Study the drawing (mm; zero at the part's minimum x, y, z) and answer. Coordinates: 2 decimals unless noted, no trailing zeros. Write each loop counter-clockwise with the first axis right and the second up, starting at its lowest first coordinate (ties: lowest second). Pieces come first, ordered by that corner, then holes. Notation, with made-up numbers: (74, 42.25) - (125, 42.25) arc R10 cw to (125, 58.25) - close; hole circle Ø1 at (57, -10.5). An arc over 180 degrees is marked (long way). One line per item, written item: value.
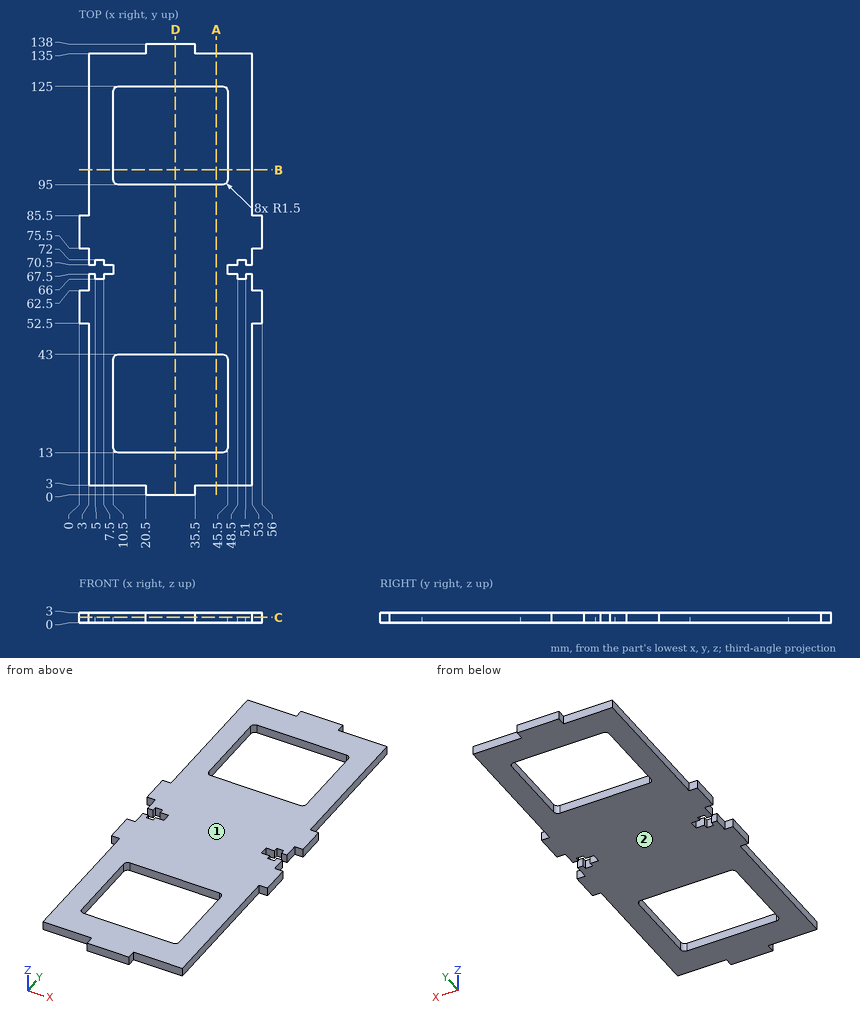
Item 1: Given pin 1 (1.5 mm diameter, centred on x = 55, z = 2, fed in from -Y); pin 2 (1.2 mm diameter, centred on x = 50.5, z = 2, fed in from -Y); pin 3 (1.5 mm diameter, centred on y = 1.5, z = 1, fed in from -X), each flat-ended and moving along its own axis, determine where each tip first touches the part or whether it passes through.
Evaluation:
pin 1: stops at y = 52.5
pin 2: stops at y = 3
pin 3: stops at x = 20.5
Item 2: Section C-C, the plane z = 1.65 is taken. Give the number of separate pieces and of enclosed holes in the cut face, then the cut area to 3 significant figures.
Evaluation:
separate pieces: 1
enclosed holes: 2
area: 4,650 mm2
Item 3: Determine the mould class of the marked faces 1 and 2 for opening direction Z: +Z half, -Z half, draft (parallel to the pull), parting line (faces both ways), or undercut.
Evaluation:
face 1: +Z half
face 2: -Z half
Item 4: Section A-A, the plane x = 42 is taken. Determine the outline of the cut face in (y, z).
Evaluation:
outline: (3, 0) - (13, 0) - (13, 3) - (3, 3) - close; (43, 0) - (95, 0) - (95, 3) - (43, 3) - close; (125, 0) - (135, 0) - (135, 3) - (125, 3) - close
Item 5: Section B-B, the plane y = 99.5 is taken. Determine the outline of the cut face in (x, z), then the cut area to 3 significant figures.
Evaluation:
outline: (3, 0) - (10.5, 0) - (10.5, 3) - (3, 3) - close; (45.5, 0) - (53, 0) - (53, 3) - (45.5, 3) - close
area: 45.0 mm2
Item 6: Section D-D, the plane x = 29.5 is taken. Determine the outline of the cut face in (y, z).
Evaluation:
outline: (0, 0) - (13, 0) - (13, 3) - (0, 3) - close; (43, 0) - (95, 0) - (95, 3) - (43, 3) - close; (125, 0) - (138, 0) - (138, 3) - (125, 3) - close
Item 7: Consider probe 1 along Y at (x, z) = (42, 1.95); probe 2 along Y at (x, z) = (32, 2.6); probe 3 along X at (y, z) = (26.5, 1.95). Determine where each line is inside the solid, lowest interval first.
Evaluation:
probe 1: y = 3 to 13, 43 to 95, 125 to 135
probe 2: y = 0 to 13, 43 to 95, 125 to 138
probe 3: x = 3 to 10.5, 45.5 to 53
